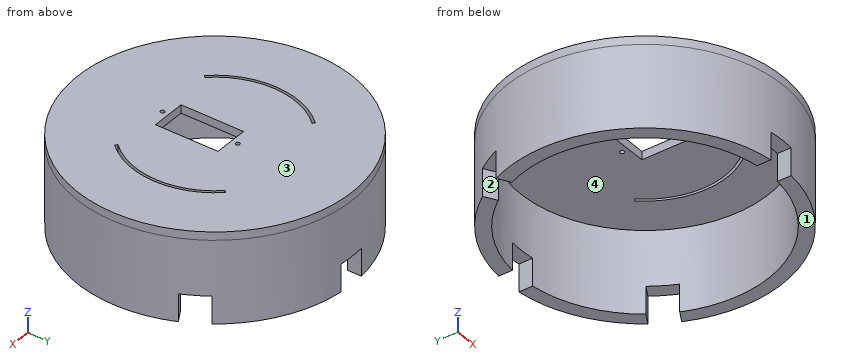
```python
from build123d import *

# Parameters (mm, degrees)
SKETCH1_R           = 50
BOSS_EXTRUDE2_DEPTH = 3
BOSS_EXTRUDE3_START = 30
SKETCH4_R           = 50
SKETCH4_R_2         = 45
BOSS_EXTRUDE3_DEPTH = 30
SKETCH6_W           = 10
SKETCH6_H           = 13.969019588
SKETCH6_H_2         = 16.825930606
CUT_EXTRUDE5_DEPTH  = 10
SKETCH2_R           = 0.75
SKETCH2_W           = 12.6
SKETCH2_H           = 22.86
CUT_EXTRUDE6_DEPTH  = 89.883910805
CUT_EXTRUDE7_DEPTH  = 10


with BuildPart() as part:
    # Sketch1 → Boss-Extrude2 (new body)
    with BuildSketch(Plane.XY):
        with Locations((0.3, 16.86)):
            Circle(SKETCH1_R)
    extrude(amount=BOSS_EXTRUDE2_DEPTH)

    # Sketch4 → Boss-Extrude3 (add)
    with BuildSketch(Plane(origin=(0, 0, 0), x_dir=(-1, 0, 0), z_dir=(0, 0, -1)).offset(BOSS_EXTRUDE3_START)):
        with Locations((-0.3, 16.86)):
            Circle(SKETCH4_R)
        with Locations((-0.3, 16.86)):
            Circle(SKETCH4_R_2, mode=Mode.SUBTRACT)
    extrude(amount=-BOSS_EXTRUDE3_DEPTH)

    # Sketch6 → Cut-Extrude5 (cut)
    with BuildSketch(Plane(origin=(0, 0, -30), x_dir=(-1, 0, 0), z_dir=(0, 0, -1))):
        Polygon((-44.927169294, 48.323775511), (-32.829643465, 41.339265717), (-37.829643465, 32.679011679), (-49.927169294, 39.663521473), align=None)
        with Locations((-0.234844245, -30.535640269)):
            Rectangle(SKETCH6_W, SKETCH6_H)
        Polygon((49.262013539, 39.776374552), (37.164487709, 32.791864758), (32.164487709, 41.452118796), (44.262013539, 48.43662859), align=None)
        with Locations((-0.234844245, 64.462731708)):
            Rectangle(SKETCH6_W, SKETCH6_H_2)
    extrude(amount=-CUT_EXTRUDE5_DEPTH, mode=Mode.SUBTRACT)

    # Sketch2 → Cut-Extrude6 (cut, through all)
    with BuildSketch(Plane(origin=(0, 0, 0), x_dir=(-1, 0, 0), z_dir=(0, 0, -1))):
        with Locations((-0.3, -2.32)):
            Circle(SKETCH2_R)
        with Locations((-0.3, 25.18)):
            Circle(SKETCH2_R)
        with Locations((-0.6, 11.43)):
            Rectangle(SKETCH2_W, SKETCH2_H)
    extrude(amount=-CUT_EXTRUDE6_DEPTH, mode=Mode.SUBTRACT)

    # Sketch7 → Cut-Extrude7 (cut)
    with BuildSketch(Plane.XY.offset(3)):
        with BuildLine():
            Line((-21.802387412, 37.145080002), (-21.065641165, 36.468910669))
            ThreePointArc((-21.065641165, 36.468910669), (-28.7, 16.86), (-21.065641165, -2.748910669))
            Line((-21.065641165, -2.748910669), (-21.802387412, -3.425080002))
            ThreePointArc((-21.802387412, -3.425080002), (-29.7, 16.86), (-21.802387412, 37.145080002))
        make_face()
        with BuildLine():
            Line((21.665641165, -2.748910669), (22.402387412, -3.425080002))
            ThreePointArc((22.402387412, -3.425080002), (30.3, 16.86), (22.402387412, 37.145080002))
            Line((22.402387412, 37.145080002), (21.665641165, 36.468910669))
            ThreePointArc((21.665641165, 36.468910669), (29.3, 16.86), (21.665641165, -2.748910669))
        make_face()
    extrude(amount=-CUT_EXTRUDE7_DEPTH, mode=Mode.SUBTRACT)


solid = part.part
```
Work out the finished part from the listing and answer in its coordinate system (mm). Face numbers are marked on the shaded views. A direction names the side the tool comes from. Round coordinates to 2 decimals unless told otherwise and drop trailing zeros. Write each loop counter-clockwise with the first axis right and the second up, starting at its lowest first coordinate (ties: lowest second). Pieces come first, ordered by that corner, then holes. Notation, with made-up numbers: (31, -25.75) - (59, -25.75) arc R37 ccw to (59, 10.25) - close; hole circle Ø5 at (-13, 44.25). An arc over 180 degrees is marked (long way). Return JSON: item names as keys, results as strings. Group by question number.
Q1. The mould has two halves that part along Y. Classify the marked faces 1 and 2: released by +Y, released by -Y, zero draft, split by the parting line, or undercut.
Q2. The part is cut by section A-A on z = -23. Write down the section's boundary in (x, y), then the cut area to 3 significant figures.
Q3. The part is cut by section D-D on z = -9. Write down the section's boundary in (x, y).
Q4. The part is cut by section B-B on y = 16.86. Write down the section's boundary in (x, z).
Q5. Find the intervals of material crossed by L1, parallel to Y at x = 0.3, z = 2.25; L2, parallel to Y at x = 0.3, z = -18.5; L3, parallel to Y at x = 0, z = 1, in increasing order.
Q6. Each of these flat-tipped pins is pushed along its axis until it touches: pin 1 Ø1.5 at (x, z) = (0.5, 1.5) entering from +Y; pin 2 Ø5 at (x, z) = (27, -9.5) entering from +Y; pin 3 Ø2 at (x, y) = (0.3, 25.18) entering from -Z. Where does it stop, or does it pass through?
Q7. The part is cut by section C-C on y = 55.5. Write down the section's boundary in (x, z), then the cut area to 4 significant figures.
Q8. For the marked faces 3 and 4, determine the directions among +Z, -Z, +X, -X, +Y, -Y from which every point of the face is accessible in a straight line to the end or side of a thin tool.
Solved:
{
 "1": {"face 1": "zero draft", "face 2": "undercut"},
 "2": {"outline": "(-45.26, 37.46) arc R50 ccw to (-4.77, -32.88) - (-4.77, -27.85) arc R45 cw to (-40.9, 34.95) - close; (-40.25, 46.12) - (-35.89, 43.6) arc R45 cw to (-4.77, 61.57) - (-4.77, 66.6) arc R50 ccw to start; (5.23, -32.9) arc R50 ccw to (45.91, 37.34) - (41.56, 34.83) arc R45 cw to (5.23, -27.87) - close; (5.23, 61.59) arc R45 cw to (36.57, 43.5) - (40.92, 46.01) arc R50 ccw to (5.23, 66.62) - close", "area": "1,290 mm²"},
 "3": {"outline": "circle Ø100 at (0.3, 16.86); hole circle Ø90 at (0.3, 16.86)"},
 "4": {"outline": "(-49.7, -30) - (-44.7, -30) - (-44.7, 0) - (-29.7, 0) - (-29.7, 3) - (-49.7, 3) - close; (-28.7, 0) - (-5.7, 0) - (-5.7, 3) - (-28.7, 3) - close; (6.9, 0) - (29.3, 0) - (29.3, 3) - (6.9, 3) - close; (30.3, 0) - (45.3, 0) - (45.3, -30) - (50.3, -30) - (50.3, 3) - (30.3, 3) - close"},
 "5": {"L1": "-33.14 to -3.07, -1.57 to 0, 22.86 to 24.43, 25.93 to 66.86", "L2": "-33.14 to -28.14, 61.86 to 66.86", "L3": "-33.14 to -3.01, -1.63 to 0, 22.86 to 24.49, 25.87 to 66.86"},
 "6": {"pin 1": "y = 66.86", "pin 2": "y = 60.61", "pin 3": "z = 0"},
 "7": {"outline": "(-31.43, -30) - (-22.76, -30) - (-22.76, 0) - (23.36, 0) - (23.36, -30) - (32.03, -30) - (32.03, 3) - (-31.43, 3) - close", "area": "710.5 mm²"},
 "8": {"face 3": "+Z, +X, -X, +Y, -Y", "face 4": "-Z"}
}
